from build123d import *

# Parameters (mm, degrees)
SKETCH1_W           = 20
SKETCH1_H           = 20
BOSS_EXTRUDE1_DEPTH = 2.5
CUT_EXTRUDE1_REACH  = 24.5
SKETCH2_R           = 1


with BuildPart() as part:
    # Sketch1 → Boss-Extrude1 (new, symmetric)
    with BuildSketch(Plane(origin=(0, 0, 0), x_dir=(1, 0, 0), z_dir=(0, 1, 0))):
        Rectangle(SKETCH1_W, SKETCH1_H)
    extrude(amount=BOSS_EXTRUDE1_DEPTH, both=True)

    # Sketch2 → Cut-Extrude1 (cut, up to next)
    with BuildSketch(Plane(origin=(10, 0, 0), x_dir=(0, 0, -1), z_dir=(1, 0, 0)), mode=Mode.PRIVATE) as cut_extrude1_sk1:
        with Locations((-8, 0)):
            Circle(SKETCH2_R)
    cut_extrude1_tool1 = extrude(cut_extrude1_sk1.sketch, amount=-CUT_EXTRUDE1_REACH, mode=Mode.PRIVATE) & part.part
    add(cut_extrude1_tool1.solids().sort_by_distance((10, 0, 8))[0], mode=Mode.SUBTRACT)


solid = part.part
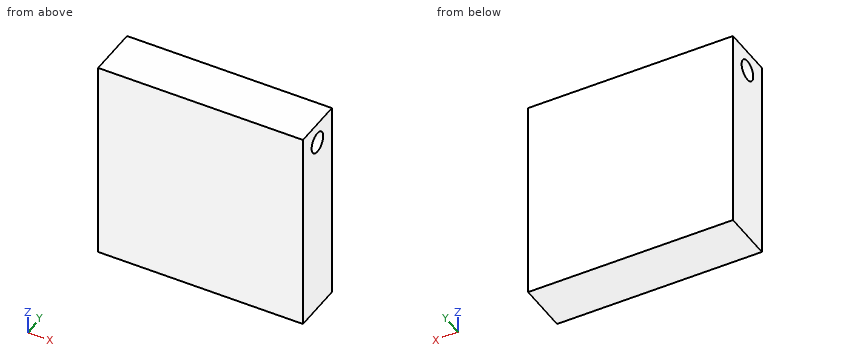
Model file for the job. Use its own axes, mm. Give positions to 0.01 mm unless a question says otherwise; leave off trailing zeros. Loops run counter-clockwise (first coordinate to the right, second up) from the corner with the lowest first, then second, coordinate; pieces in that order, holes last. Notation, with made-up numbers: (-32, 78.25) -> (-12, 78.25) arc R15 cw to (-12, 84.25) -> close; hole circle Ø9 at (-23.75, 78). An arc over 180 degrees is marked (long way). Use a Markdown table: item, result. Add a question column.
(1) Slice it at C-C on x = -8.5. List the corners of the cut face in (y, z).
(2) Wall check: line 1 along Y through (x, z) = (-5.5, 8); line 2 along Z through (x, y) = (-0.75, 0.5); line 3 along Z through (x, y) = (6, 0.25). Give the ranges that are in metal, low to high.
(3) Slice it at A-A on z = 8. List the corners of the cut face in (x, y), and give its area (3 significant figures).
(4) Slice it at B-B on y = 0. List the corners of the cut face in (x, z), and give its area (3 significant figures).
Filled sheet:
| question | item | result |
|---|---|---|
| 1 | outline | (-2.5, -10) -> (2.5, -10) -> (2.5, 10) -> (-2.5, 10) -> close; hole circle Ø2 at (0, 8) |
| 2 | line 1 | -2.5 to -1, 1 to 2.5 |
| 2 | line 2 | -10 to 7.13, 8.87 to 10 |
| 2 | line 3 | -10 to 7.03, 8.97 to 10 |
| 3 | outline | (-10, -2.5) -> (10, -2.5) -> (10, -1) -> (-10, -1) -> close; (-10, 1) -> (10, 1) -> (10, 2.5) -> (-10, 2.5) -> close |
| 3 | area | 60.0 mm2 |
| 4 | outline | (-10, -10) -> (10, -10) -> (10, 7) -> (-10, 7) -> close; (-10, 9) -> (10, 9) -> (10, 10) -> (-10, 10) -> close |
| 4 | area | 360 mm2 |
